```python
from build123d import *

# Parameters (mm, degrees)
SKETCH_W        = 20.5
SKETCH_H        = 20.5
PAD_DEPTH       = 5
SKETCH001_W     = 26.5
SKETCH001_H     = 26.5
SKETCH001_W_2   = 20.5
SKETCH001_H_2   = 20.5
PAD001_DEPTH    = 10
CHAMFER_SIZE    = 4
CHAMFER001_SIZE = 1
CHAMFER002_SIZE = 1.8
CHAMFER003_SIZE = 2
SKETCH003_R     = 3


with BuildPart() as part:
    # Sketch → Pad (new body)
    with BuildSketch(Plane.XY):
        Polygon((7.25, -15), (15, -7.25), (15, 27.75), (7.25, 35.5), (-27.75, 35.5), (-35.5, 27.75), (-35.5, -7.25), (-27.75, -15), align=None)
        with Locations((-10.25, 10.25)):
            Rectangle(SKETCH_W, SKETCH_H, mode=Mode.SUBTRACT)
    extrude(amount=PAD_DEPTH)

    # Sketch001 (on Face14 of Pad) → Pad001 (join)
    with BuildSketch(Plane.XY.offset(5)):
        with Locations((-10.25, 10.25)):
            Rectangle(SKETCH001_W, SKETCH001_H)
        with Locations((-10.25, 10.25)):
            Rectangle(SKETCH001_W_2, SKETCH001_H_2, mode=Mode.SUBTRACT)
    extrude(amount=PAD001_DEPTH)

    # Chamfer
    chamfer_edges = [part.edges().sort_by_distance(p)[0] for p in [
        (-10.25, -3, 5),
        (3, 10.25, 5),
        (-10.25, 23.5, 5),
        (-23.5, 10.25, 5),
    ]]
    chamfer(chamfer_edges, length=CHAMFER_SIZE)

    # Chamfer001
    chamfer001_edges = [part.edges().sort_by_distance(p)[0] for p in [
        (0, 10.25, 15),
        (-10.25, 0, 15),
        (-20.5, 10.25, 15),
        (-10.25, 20.5, 15),
    ]]
    chamfer(chamfer001_edges, length=CHAMFER001_SIZE)

    # Chamfer002
    chamfer002_edges = [part.edges().sort_by_distance(p)[0] for p in [
        (3, 10.25, 15),
        (-10.25, 23.5, 15),
        (-23.5, 10.25, 15),
        (-10.25, -3, 15),
    ]]
    chamfer(chamfer002_edges, length=CHAMFER002_SIZE)

    # Chamfer003
    chamfer003_edges = [part.edges().sort_by_distance(p)[0] for p in [
        (15, 10.25, 5),
        (11.125, 31.625, 5),
        (-10.25, 35.5, 5),
        (-31.625, 31.625, 5),
        (-35.5, 10.25, 5),
        (-31.625, -11.125, 5),
        (-10.25, -15, 5),
        (11.125, -11.125, 5),
    ]]
    chamfer(chamfer003_edges, length=CHAMFER003_SIZE)

    # SubtractivePipe: sweep along a path in Sketch002
    with BuildLine(Plane(origin=(0, 0, 0), x_dir=(1, 0, 0), z_dir=(0, 0, -1))) as subtractivepipe_path:
        Line((-27.5, -23.964466), (-27.5, 4.464466))
        Line((-27.5, 4.464466), (-23.964466, 8))
        Line((-23.964466, 8), (3.464466, 8))
        Line((3.464466, 8), (7, 4.464466))
        Line((7, 4.464466), (7, -23.964466))
        Line((7, -23.964466), (3.464466, -27.5))
        Line((3.464466, -27.5), (-23.964466, -27.5))
        Line((-23.964466, -27.5), (-27.5, -23.964466))
    # Sketch003 → SubtractivePipe (sweep, cut)
    with BuildSketch(Plane.XZ):
        with Locations((-27.5, 0)):
            Circle(SKETCH003_R)
    sweep(path=subtractivepipe_path.line, transition=Transition.RIGHT, mode=Mode.SUBTRACT)


solid = part.part
```
For this review, take the finished solid that the model builds, in its own axes (mm). A direction names the side the tool comes from. Round coordinates to 2 decimals unless told otherwise and drop trailing zeros. Loops run counter-clockwise (first coordinate to the right, second up) from the corner with the lowest first, then second, coordinate; pieces in that order, holes last.
Q1. Insertion check: pin 1 Ø2 at (y, z) = (10.5, 11) entering from +X; pin 2 Ø2 at (x, y) = (-1.5, -3) entering from +Z; pin 3 Ø4 at (x, z) = (-8, 10) entering from -Y. Each pin has a flat end and moves straight along its axis. Give the tip position at first contact, or say it passes through.
Result sheet:
pin 1: stops at x = 3
pin 2: stops at z = 14.2
pin 3: stops at y = -4
Q2. Add section C-C on z = 8. Write out the cut boundary in (x, y).
Result sheet:
outline: (-24.5, -4) - (4, -4) - (4, 24.5) - (-24.5, 24.5) - close; hole (-20.5, 0) - (0, 0) - (0, 20.5) - (-20.5, 20.5) - close
Q3. Machinability: for faces 1 (the face through (-23.5, 10, 11)), 2 (the face through (-10, 0, 7)), 3 (the face through (3, 10, 11)), 4 (the face through (-10, -8, 3)), which of the approach directions +Z, -Z, +X, -X, +Y, -Y give a long, thin tool a straight path to every point of the face, cutting with its end or side? Answer none if there is none.
Result sheet:
face 1: +Z, -X, +Y, -Y
face 2: +Z, -Z
face 3: +Z, +X, +Y, -Y
face 4: -Z
Q4. Add section B-B on y = 9. Write out the cut boundary in (x, z).
Result sheet:
outline: (-35.5, 0) - (-30.5, 0) arc R3 cw to (-24.5, 0) - (-20.5, 0) - (-20.5, 14) - (-21.5, 15) - (-21.7, 15) - (-23.5, 13.2) - (-23.5, 9) - (-27.5, 5) - (-33.5, 5) - (-35.5, 3) - close; (0, 0) - (4, 0) arc R3 cw to (10, 0) - (15, 0) - (15, 3) - (13, 5) - (7, 5) - (3, 9) - (3, 13.2) - (1.2, 15) - (1, 15) - (0, 14) - close
Q5. To check wall thickness, follow line 1 along X through (y, z) = (12, 1.25); line 2 along Y through (x, z) = (-10.5, 10.25); line 3 along Y through (x, z) = (-14, 1.75). State the ranges of each line that lie inside material, in increasing order.
Result sheet:
line 1: x = -35.5 to -30.23, -24.77 to -20.5, 0 to 4.27, 9.73 to 15
line 2: y = -3 to 0, 20.5 to 23.5
line 3: y = -15 to -10.44, -5.56 to 0, 20.5 to 25.06, 29.94 to 35.5
Q6. Mouldability with a two-part tool opening along Y and no side actions: class faces 5 (the face through (-35.5, 10, 1)), 6 (the face through (11.18, 31.57, 1.48)), 7 (the face through (-26.45, 26.38, 2.84)) as +Y half, -Y half, draft (parallel to the pull), parting line (faces both ways), or undercut.
Result sheet:
face 5: draft
face 6: +Y half
face 7: undercut
Q7. Add section A-A on x = -5. Write out the cut boundary in (y, z).
Result sheet:
outline: (-15, 0) - (-11, 0) arc R3 cw to (-5, 0) - (0, 0) - (0, 14) - (-1, 15) - (-1.2, 15) - (-3, 13.2) - (-3, 9) - (-7, 5) - (-13, 5) - (-15, 3) - close; (20.5, 0) - (24.5, 0) arc R3 cw to (30.5, 0) - (35.5, 0) - (35.5, 3) - (33.5, 5) - (27.5, 5) - (23.5, 9) - (23.5, 13.2) - (21.7, 15) - (21.5, 15) - (20.5, 14) - close
